Input: part model. Units: mm. Frame: model coordinates. Face numbers are marked on the shaded views. A direction names the side the tool comes from. Coordinates: 2 decimals unless noted, no trailing zeros. Order: outer loops, then holes, each group sorted by start corner. A loop starts at its lowest first (then second) coordinate and runs counter-clockwise, first axis right, second up. Notation, with made-up numbers: (12, 32) - (49, 32) arc R26 ccw to (49, 57) - close; hole circle Ø4 at (-18.5, 7). An arc over 180 degrees is marked (long way). One line per question, with ' | ' between items.
from build123d import *

# Parameters (mm, degrees)
SKETCH_W        = 38
SKETCH_H        = 27
SKETCH_R        = 1.65
PAD_DEPTH       = 3
SKETCH001_R     = 5
PAD001_DEPTH    = 38
SKETCH002_R     = 1.6
POCKET_DEPTH    = 19.894216
SKETCH004_R     = 1.25
POCKET002_DEPTH = 20.001
SKETCH005_R     = 3.25
POCKET003_DEPTH = 16.894216
CHAMFER_SIZE    = 1
CHAMFER001_SIZE = 1


with BuildPart() as part:
    # Sketch → Pad (new body)
    with BuildSketch(Plane.XY):
        Rectangle(SKETCH_W, SKETCH_H)
        with Locations((-13, -10)):
            Circle(SKETCH_R, mode=Mode.SUBTRACT)
        with Locations((-13, 10)):
            Circle(SKETCH_R, mode=Mode.SUBTRACT)
        with Locations((13, 10)):
            Circle(SKETCH_R, mode=Mode.SUBTRACT)
        with Locations((13, -10)):
            Circle(SKETCH_R, mode=Mode.SUBTRACT)
    extrude(amount=PAD_DEPTH)

    # Sketch001 (on Face2 of Pad) → Pad001 (join)
    with BuildSketch(Plane.YZ.offset(19)):
        with BuildLine():
            ThreePointArc((7.5, 12.393216), (0, 19.893216), (-7.5, 12.393216))
            Line((-7.5, 12.393216), (-13.5, 0))
            Line((-13.5, 0), (13.5, 0))
            Line((7.5, 12.393216), (13.5, 0))
        make_face()
        with Locations((0, 12.393216)):
            Circle(SKETCH001_R, mode=Mode.SUBTRACT)
    extrude(amount=-PAD001_DEPTH)

    # Sketch002 (on Face4 of Pad001) → Pocket (cut, through all)
    with BuildSketch(Plane(origin=(0, 0, 0), x_dir=(1, 0, 0), z_dir=(0, 0, -1))):
        with Locations((13, 10)):
            Circle(SKETCH002_R)
        with Locations((-13, 10)):
            Circle(SKETCH002_R)
        with Locations((-13, -10)):
            Circle(SKETCH002_R)
        with Locations((13, -10)):
            Circle(SKETCH002_R)
    extrude(amount=-POCKET_DEPTH, mode=Mode.SUBTRACT)

    # Sketch004 → Pocket002 (cut, through all)
    with BuildSketch(Plane.XY.offset(20)):
        Circle(SKETCH004_R)
    extrude(amount=-POCKET002_DEPTH, mode=Mode.SUBTRACT)

    # Sketch005 (on Face19 of Pocket002) → Pocket003 (cut, through all)
    with BuildSketch(Plane.XY.offset(3)):
        with Locations((-13, 10)):
            Circle(SKETCH005_R)
        with Locations((13, 10)):
            Circle(SKETCH005_R)
        with Locations((13, -10)):
            Circle(SKETCH005_R)
        with Locations((-13, -10)):
            Circle(SKETCH005_R)
    extrude(amount=POCKET003_DEPTH, mode=Mode.SUBTRACT)

    # Chamfer
    chamfer_edges = [part.edges().sort_by_distance(p)[0] for p in [
        (19, -5, 12.393216),
    ]]
    chamfer(chamfer_edges, length=CHAMFER_SIZE)

    # Chamfer001
    chamfer001_edges = [part.edges().sort_by_distance(p)[0] for p in [
        (-19, -5, 12.393216),
    ]]
    chamfer(chamfer001_edges, length=CHAMFER001_SIZE)


solid = part.part
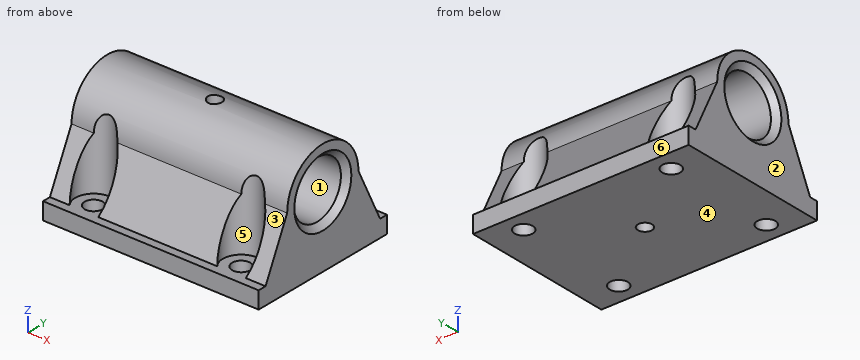
Item 1: Contact query for flat-ended pins moving along their axis: P1, Ø1, axis at x = 10, z = 4, coming from the +Y side; P2, Ø3, axis at x = 14, y = -7, coming from the +Z side; P3, Ø6, axis at x = 0, y = -9, coming from the +Z side. Output: stop coordinate, or through.
Data:
P1: y = 11.81 | P2: z = 17.49 | P3: z = 16.89
Item 2: Section D-D on z = 4.5. Return the cut outline in (x, y), and give its area (3 significant figures).
Data:
outline: (-19, -11.32) - (-15.97, -11.32) arc R3.25 cw (long way) to (-10.03, -11.32) - (10.03, -11.32) arc R3.25 cw (long way) to (15.97, -11.32) - (19, -11.32) - (19, 11.32) - (15.97, 11.32) arc R3.25 cw (long way) to (10.03, 11.32) - (-10.03, 11.32) arc R3.25 cw (long way) to (-15.97, 11.32) - (-19, 11.32) - close; hole circle Ø2.5 at (0, 0) | area: 756 mm^2
Item 3: Section A-A on x = 13. Return the cut outline in (y, z).
Data:
outline: (-13.5, 0) - (-11.6, 0) - (-11.6, 3) - (-13.5, 3) - close; (-8.4, 0) - (8.4, 0) - (8.4, 3) - (6.75, 3) - (6.75, 15.66) arc R7.5 ccw to (-6.75, 15.66) - (-6.75, 3) - (-8.4, 3) - close; (11.6, 0) - (13.5, 0) - (13.5, 3) - (11.6, 3) - close; hole circle Ø10 at (0, 12.39)
Item 4: Section B-B on x = -3.5. Return the cut outline in (y, z), and give its area (3 significant figures).
Data:
outline: (-13.5, 0) - (13.5, 0) - (13.5, 3) - (12.05, 3) - (7.5, 12.39) arc R7.5 ccw to (-7.5, 12.39) - (-12.05, 3) - (-13.5, 3) - close; hole circle Ø10 at (0, 12.39) | area: 274 mm^2
Item 5: Section C-C on y = 10. Return the cut outline in (x, z).
Data:
outline: (-19, 0) - (-14.6, 0) - (-14.6, 3) - (-16.25, 3) - (-16.25, 7.23) - (-19, 7.23) - close; (-11.4, 0) - (11.4, 0) - (11.4, 3) - (9.75, 3) - (9.75, 7.23) - (-9.75, 7.23) - (-9.75, 3) - (-11.4, 3) - close; (14.6, 0) - (19, 0) - (19, 7.23) - (16.25, 7.23) - (16.25, 3) - (14.6, 3) - close
Item 6: Access query for the marked faces 5 and 6. Directions: +Z, -Z, +X, -X, +Y, -Y. A direction counts if a zero-diameter tool reaches every point of the face in a straight line with its end or side. Return the directions, or none.
Data:
face 5: +Z | face 6: +Z, -Z, +X, -X, +Y
Item 7: Ray query, line 1 (Y direction, x = 13, z = 0.8); line 2 (X direction, y = -10, z = 1.5); line 3 (X direction, y = -7.25, z = 11.25). Return the intervals inside material, ascending.
Data:
line 1: -13.5 to -11.6, -8.4 to 8.4, 11.6 to 13.5 | line 2: -19 to -14.6, -11.4 to 11.4, 14.6 to 19 | line 3: -19 to -14.73, -11.27 to 11.27, 14.73 to 19
Item 8: Draft query along Z for the marked faces 1, 2, 3 and 4. Return one class per face: released by +Z, released by -Z, zero draft, split by the parting line, or undercut.
Data:
face 1: undercut | face 2: zero draft | face 3: released by +Z | face 4: released by -Z
